Design review of the part built by this model. Coordinates are the model's own, in mm. A direction names the side the tool comes from. Round coordinates to 2 decimals unless told otherwise and drop trailing zeros. Order: outer loops, then holes, each group sorted by start corner. A loop starts at its lowest first (then second) coordinate and runs counter-clockwise, first axis right, second up. Notation, with made-up numbers: M -34,4 L -10,4 A16 ccw -10,32 Z; hole C 28.25,42 d9. An arc over 180 degrees is marked long. Write item = value, one per line. Start each with the question number.
```python
from build123d import *

# Parameters (mm, degrees)
F3_DEPTH = 18.25
F5_DEPTH = 29


with BuildPart() as f1:
    # F0 (on Front) → F1 (revolve)
    with BuildSketch(Plane.XZ):
        Polygon((8, 0), (0, 0), (0, -2), (9.769411, -2), (13.269411, 26.5), (14.54639, 26.5), (15.40639, 37.25), (13.4, 37.25), (12.7, 28.5), (11.5, 28.5), align=None)
    revolve(axis=Axis((0, 0, 14.25), (0, 0, 1)))

    # F2 (on face) → F3 (cut)
    with BuildSketch(Plane(origin=(0, 0, 26.5), x_dir=(1, 0, 0), z_dir=(0, 0, -1))):
        Polygon((-21.099057, 0), (-20.108491, 0), (0, 0), (0, 20.207549), (-21.099057, 20.207549), align=None)
        Polygon((0, 0), (-20.108491, 0), (-20.108491, -19.117925), (20.306604, -19.117925), (20.306604, 0), align=None)
    extrude(amount=F3_DEPTH, mode=Mode.SUBTRACT)

    # F4 (on face) → F5 (cut)
    with BuildSketch(Plane.XY.offset(37.25)):
        Polygon((25.364828, 31.607275), (-31.607275, 31.607275), (25.364828, -25.364828), align=None)
    extrude(amount=-F5_DEPTH, mode=Mode.SUBTRACT)


solid = f1.part
```
(1) Consider section D-D, the plane z = 25. Write out the cut boundary in (x, y), then the cut area to 3 significant figures.
(2) For faces 5 (the face through (0, -11, 18)), 6 (the face through (-10.825, -10.359, 31.95)), 7 (the face through (-8.3, -8.2, 28.5)), list the 3-axis set-ups (+Z, -Z, +X, -X, +Y, -Y) from which the entire face can be reached by the end or side of a thin tool; tool diameter is ignored.
(3) For line 1 along Y through (x, z) = (3.5, 7); line 2 along Z through (x, y) = (-4.25, -6); line 3 along Z through (x, y) = (-3.5, 9), list the stretches that pass through material, from the lowest coordinate up. Write a range as [from, to].
(4) Consider section A-A, the plane y = 0. Write out the cut boundary in (x, z), then the cut area to 3 significant figures.
(5) Insertion check: pin 1 (3.5 mm diameter, centred on y = -11.5, z = 17, fed in from -X); pin 2 (6.5 mm diameter, centred on x = -7, y = -6, fed in from +Z); pin 3 (2 mm diameter, centred on x = -8, y = -10, fed in from -Z); pin 4 (8 mm diameter, centred on y = 8, z = 15, fed in from +X). Each pin has a flat end and moves straight along its axis. Give the tip position at first contact, or say it passes through.
(6) Draft analysis for pull direction Y (two halves, no side actions). For faces 1 (the face through (8.6, -8.6, 22.8)), 2 (the face through (0, 0, -2)), 3 (the face through (0, 0, 0)), 4 (the face through (4.788, -9.206, 2.95)), state which applies: pulls with the +Y half, pulls with the -Y half, needs draft (parallel to the pull), parting line crosses it, or undercut.
(7) Consider section C-C, the plane z = 3.5. Write out the cut boundary in (x, y), then the cut area to 3 significant figures.
(8) Consider section B-B, the plane z = 14. Write out the cut boundary in (x, y).
Completed:
q1.outline = M 0,-13.09 A13.09 ccw 9.25,-9.25 L 7.83,-7.83 A11.07 cw 0,-11.07 Z
q1.area = 19.1 mm2
q2.face_5 = -X, +Y, -Y
q2.face_6 = -Z
q2.face_7 = +Z
q3.line_1 = [-10.3, -8.14], [8.14, 10.3]
q3.line_2 = [-2, 0]
q3.line_3 = [-2, 8.25]
q4.outline = M -15.41,37.25 L -14.55,26.5 L -11.25,26.5 L -11.5,28.5 L -12.7,28.5 L -13.4,37.25 Z; M -11.03,8.25 L -9.77,-2 L 9.77,-2 L 11.03,8.25 L 9.01,8.25 L 8,0 L -8,0 L -9.01,8.25 Z
q4.area = 96.9 mm2
q5.pin_1 = 0
q5.pin_2 = 28.5
q5.pin_3 = 26.5
q5.pin_4 = through
q6.face_1 = pulls with the +Y half
q6.face_2 = needs draft
q6.face_3 = undercut
q6.face_4 = parting line crosses it
q7.outline = C 0,0 d20.89; hole C 0,0 d16.86
q7.area = 119 mm2
q8.outline = M 0,-11.73 A11.73 ccw 8.3,-8.3 L 6.87,-6.87 A9.72 cw 0,-9.72 Z
